Source: CAD feature listing. Evaluate the final solid. Frame: model axes, mm. A direction names the side the tool comes from. Coordinates: 2 decimals unless noted, no trailing zeros. Write each loop counter-clockwise with the first axis right and the second up, starting at its lowest first coordinate (ties: lowest second). Pieces come first, ordered by that corner, then holes. Notation, with made-up numbers: (39, 67) - (93, 67) arc R22 ccw to (93, 104) - close; hole circle Ø3 at (-5, 64). An arc over 180 degrees is marked (long way). One line per item, written item: value.
from build123d import *

# Parameters (mm, degrees)
SKETCH_R        = 6.25
PAD_DEPTH       = 1.5
SKETCH001_R     = 4.6
PAD001_DEPTH    = 10
SKETCH002_R     = 2
PAD002_DEPTH    = 2
SKETCH003_R     = 1
PAD003_DEPTH    = 4.5
SKETCH006_R     = 4.75
SKETCH006_R_2   = 3.75
PAD004_DEPTH    = 11.5
SKETCH007_R     = 2
PAD005_DEPTH    = 5.5
SKETCH004_R     = 0.75
POCKET_DEPTH    = 29.501
SKETCH008_R     = 1
PAD006_DEPTH    = 5.5
SKETCH009_R     = 1
POCKET001_DEPTH = 3.75
SKETCH010_R     = 6.5
SKETCH010_R_2   = 4.7
PAD007_DEPTH    = 0.5
SKETCH011_R     = 1
PAD008_DEPTH    = 0.5


with BuildPart() as part:
    # Sketch → Pad (new body)
    with BuildSketch(Plane.XY):
        Circle(SKETCH_R)
    extrude(amount=PAD_DEPTH)

    # Sketch001 (on Face2 of Pad) → Pad001 (join)
    with BuildSketch(Plane(origin=(0, 0, 0), x_dir=(1, 0, 0), z_dir=(0, 0, -1))):
        Circle(SKETCH001_R)
    extrude(amount=PAD001_DEPTH)

    # Sketch002 (on Face5 of Pad001) → Pad002 (join)
    with BuildSketch(Plane(origin=(0, 0, -10), x_dir=(1, 0, 0), z_dir=(0, 0, -1))):
        Circle(SKETCH002_R)
    extrude(amount=PAD002_DEPTH)

    # Sketch003 (on Face7 of Pad002) → Pad003 (join)
    with BuildSketch(Plane(origin=(0, 0, -12), x_dir=(1, 0, 0), z_dir=(0, 0, -1))):
        Circle(SKETCH003_R)
    extrude(amount=PAD003_DEPTH)

    # Sketch006 → Pad004 (join)
    with BuildSketch(Plane.XY.offset(1.5)):
        Circle(SKETCH006_R)
        Circle(SKETCH006_R_2, mode=Mode.SUBTRACT)
    extrude(amount=PAD004_DEPTH)

    # Sketch007 (on Face11 of Pad004) → Pad005 (join)
    with BuildSketch(Plane.XY.offset(1.5)):
        Circle(SKETCH007_R)
    extrude(amount=PAD005_DEPTH)

    # Sketch004 (on Face9 of Pad003) → Pocket (cut, through all)
    with BuildSketch(Plane(origin=(0, 0, -16.5), x_dir=(1, 0, 0), z_dir=(0, 0, -1))):
        Circle(SKETCH004_R)
    extrude(amount=-POCKET_DEPTH, mode=Mode.SUBTRACT)

    # Sketch008 → Pad006 (join, symmetric)
    with BuildSketch(Plane.XZ):
        with Locations((0, 8)):
            Circle(SKETCH008_R)
    extrude(amount=PAD006_DEPTH, both=True)

    # Sketch009 → Pocket001 (cut, symmetric)
    with BuildSketch(Plane.XZ):
        with Locations((0, 8)):
            Circle(SKETCH009_R)
    extrude(amount=POCKET001_DEPTH, both=True, mode=Mode.SUBTRACT)

    # Sketch010 (on Face2 of Pocket001) → Pad007 (join)
    with BuildSketch(Plane(origin=(0, 0, 0), x_dir=(1, 0, 0), z_dir=(0, 0, -1))):
        Circle(SKETCH010_R)
        Circle(SKETCH010_R_2, mode=Mode.SUBTRACT)
    extrude(amount=PAD007_DEPTH)

    # Sketch011 → Pad008 (join)
    with BuildSketch(Plane.XY):
        with BuildLine():
            Line((6.184658, 2), (13.184658, 2))
            ThreePointArc((13.184658, -2), (15.184658, 0), (13.184658, 2))
            Line((6.184658, -2), (13.184658, -2))
            ThreePointArc((6.184658, -2), (6.5, 0), (6.184658, 2))
        make_face()
        with Locations((13.184658, 0)):
            Circle(SKETCH011_R, mode=Mode.SUBTRACT)
    extrude(amount=-PAD008_DEPTH)


solid = part.part
1) Section query B-B on y = 0. State how many separate pieces and enclosed holes the cut face has, then the cut area to 3 significant figures.
Values found:
separate pieces: 3
enclosed holes: 0
area: 143 mm2
2) Section query C-C on z = -2.25. Output: boundary loops of the cut face in (x, y), then the cut area to 3 significant figures.
Values found:
outline: circle Ø9.2 at (0, 0); hole circle Ø1.5 at (0, 0)
area: 64.7 mm2
3) Contact query for flat-ended pins moving along their axis: P1, Ø2, axis at x = 10, z = 0, coming from the -Y side; P2, Ø1.6, axis at x = -0.5, z = 8, coming from the -Y side; P3, Ø2, axis at x = 2, z = -6.5, coming from the +Y side. Output: stop coordinate, or through.
Values found:
P1: y = -2
P2: y = -5.5
P3: y = 4.49
4) Reachability of faces 1 (the flat face through (0, -5.5, 8)), 2 (the cylindrical face through (-3.65, 2.8, -4.93)), 3 (the flat face through (0, 3.75, 8)), 4 (the cylindrical face through (-1, -5, 8)) from +Z, -Z, +X, -X, +Y, -Y: full face, straight path, thin tool, end or side. Return the list, or none.
Values found:
face 1: +Z, +X, -X, -Y
face 2: -Z
face 3: none
face 4: -Y
5) Section query A-A on z = 8. Output: boundary loops of the cut face in (x, y), then the cut area to 3 significant figures.
Values found:
outline: (-1, -5.5) - (1, -5.5) - (1, -4.64) arc R4.75 ccw to (1, 4.64) - (1, 5.5) - (-1, 5.5) - (-1, 4.64) arc R4.75 ccw to (-1, -4.64) - close; hole (-1, -3.75) - (1, -3.75) - (1, -3.61) arc R3.75 ccw to (1, 3.61) - (1, 3.75) - (-1, 3.75) - (-1, 3.61) arc R3.75 ccw to (-1, -3.61) - close
area: 29.7 mm2
6) Draft query along Z for faces 5 (the flat face through (0, -3.75, 8)), 6 (the cylindrical face through (-6.495, -0.257, -0.246)), 7 (the flat face through (1, 2, -10)). Return one class per face: released by +Z, released by -Z, zero draft, split by the parting line, or undercut.
Values found:
face 5: undercut
face 6: zero draft
face 7: released by -Z
7) Material intervals for line 1 (Y direction, x = 0, z = -5); line 2 (Y direction, x = 0, z = 10); line 3 (Z direction, x = -3.25, y = -5.5), sorted ascending.
Values found:
line 1: -4.6 to -0.75, 0.75 to 4.6
line 2: -4.75 to -3.75, 3.75 to 4.75
line 3: -0.5 to 0
